from build123d import *

# Parameters (mm, degrees)
SKETCH1_R           = 3.3734375
BOSS_EXTRUDE1_DEPTH = 6.35


with BuildPart() as part:
    # Sketch1 → Boss-Extrude1 (new body)
    with BuildSketch(Plane(origin=(0, 0, 0), x_dir=(1, 0, 0), z_dir=(0, 1, 0))):
        Polygon((1016, 406.4), (1066.8, 406.4), (1066.8, 0), (0, 0), (0, 406.4), (50.8, 406.4), (50.8, 530.225), (234.95, 530.225), (234.95, 676.275), (831.85, 676.275), (831.85, 530.225), (1016, 530.225), align=None)
        with Locations((22.225, 92.075)):
            Circle(SKETCH1_R, mode=Mode.SUBTRACT)
        with Locations((1044.575, 92.075)):
            Circle(SKETCH1_R, mode=Mode.SUBTRACT)
        with Locations((22.225, 295.275)):
            Circle(SKETCH1_R, mode=Mode.SUBTRACT)
        with Locations((1044.575, 295.275)):
            Circle(SKETCH1_R, mode=Mode.SUBTRACT)
    extrude(amount=BOSS_EXTRUDE1_DEPTH)


solid = part.part
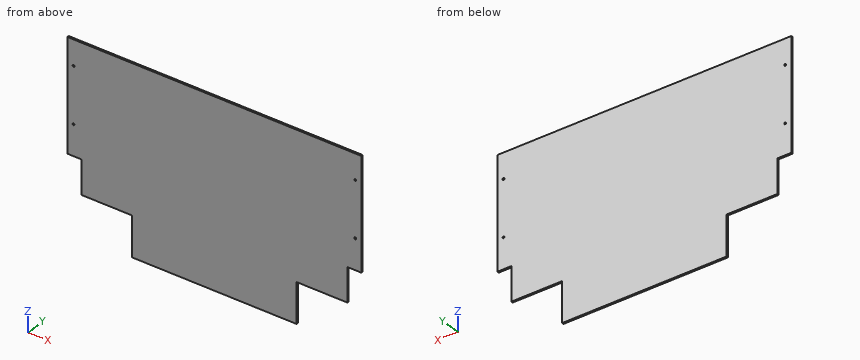
Could you check a few things on this model? Use its own coordinates, in mm. Give positions to 0.01 mm unless a question says otherwise; leave off trailing zeros. Order: outer loops, then holes, each group sorted by start corner. A loop starts at its lowest first (then second) coordinate and runs counter-clockwise, first axis right, second up. Notation, with made-up numbers: (45, -16) -> (53, -16) arc R15 cw to (53, -10) -> close; hole circle Ø2 at (67.25, -22). An arc over 180 degrees is marked (long way). Return JSON: item names as keys, results as strings.
1. Imagine slicing it at B-B on y = 2.25. List the corners of the cut face in (x, z) for me (3 decimals).
Answer list:
{"outline": "(0, -406.4) -> (50.8, -406.4) -> (50.8, -530.225) -> (234.95, -530.225) -> (234.95, -676.275) -> (831.85, -676.275) -> (831.85, -530.225) -> (1016, -530.225) -> (1016, -406.4) -> (1066.8, -406.4) -> (1066.8, 0) -> (0, 0) -> close; hole circle Ø6.747 at (22.225, -295.275); hole circle Ø6.747 at (22.225, -92.075); hole circle Ø6.747 at (1044.575, -295.275); hole circle Ø6.747 at (1044.575, -92.075)"}
2. I need wall thicknesses on line 1 (X direction, y = 2, z = -91); line 2 (X direction, y = 1.25, z = -431); line 3 (Z direction, x = 206, y = 4) (3 decimals). Which ranges of each line are inside material? Lowest first, please. Write a range as from..to.
Answer list:
{"line 1": "x = 0..19.03, 25.42..1041.38, 1047.77..1066.8", "line 2": "x = 50.8..1016", "line 3": "z = -530.225..0"}
3. For pin 1 Ø1.9 at (x, y) = (1031.5, 4.5) entering from -Z; pin 2 Ø3 at (y, z) = (4, -480.5) entering from -X; pin 3 Ø1 at (y, z) = (2.5, -535) entering from -X, each with a flat end and sliding along its axis, tell me the tip position at first contact or that it passes through.
Answer list:
{"pin 1": "stops at z = -406.4", "pin 2": "stops at x = 50.8", "pin 3": "stops at x = 234.95"}
4. Imagine slicing it at A-A on z = -601. List the corners of the cut face in (x, y) for me.
Answer list:
{"outline": "(234.95, 0) -> (831.85, 0) -> (831.85, 6.35) -> (234.95, 6.35) -> close"}
5. Imagine slicing it at C-C on x = 929. List the corners of the cut face in (y, z) for me (3 decimals).
Answer list:
{"outline": "(0, -530.225) -> (6.35, -530.225) -> (6.35, 0) -> (0, 0) -> close"}
